Autodesk Inventor part; units mm, degrees
ref_plane "YZ Plane" through (0, 0, 0) normal (1, 0, 0) x (0, 1, 0)
ref_plane "XY Plane" through (0, 0, 0) normal (0, 0, 1) x (1, 0, 0)
sketch "Sketch1" plane through (0, 0, 0) normal (0, 1, 0) x (-1, 0, 0)
  line L0 (25.9, 0) -> (-25.9, 0)
  line L1 (0, -25.9) -> (0, 25.9)
  circle A0 centre (0, 0) radius 18.5 construction
  circle A1 centre (0, 0) radius 13 construction
  dimension "d0" = 37
  dimension "d1" = 26
sketch "Sketch2" plane through (0, 0, 0) normal (0, 1, 0) x (-1, 0, 0)
  line L0 (29.4, 0) -> (-29.4, 0)
  line L1 (0, -36.8) -> (0, 73.8)
  line L2 (-21, 58) -> (-21, -21)
  line L3 (-21, -21) -> (21, -21)
  line L4 (21, -21) -> (21, 58)
  line L5 (-21, 58) -> (21, 58)
  point P0 (0, 0)
  dimension "d3" = 42
  dimension "d29" = 21
  dimension "d30" = 58
extrude "Extrusion1" add sketch "Sketch2" along normal blind 7
sketch "Sketch6" plane through (0, 0, 0) normal (0, 1, 0) x (-1, 0, 0)
  line L0 (21, -21) -> (-21, -21)
  line L1 (21, 58) -> (21, -21)
  line L2 (-21, -21) -> (21, -21)
  line L3 (21, -21) -> (21, 58)
  line L4 (-21, 58) -> (-21, -21)
  line L5 (29.4, 0) -> (-29.4, 0)
  line L6 (0, -36.3) -> (0, 70.8)
  arc A0 (-16, 0) -> (16, 0) centre (0, 0) ccw
  line L7 (16, 0) -> (16, 58)
  line L8 (21, 58) -> (-21, 58)
  line L9 (16, 58) -> (21, 58)
  line L10 (-16, 0) -> (-16, 58)
  line L11 (-16, 58) -> (-21, 58)
  point P0 (-17.3617, -21)
  dimension "d18" = 32
extrude "Extrusion5" add sketch "Sketch6" against normal blind 5.5 contours L0 L6 A0 L5 L1 | L0 L4 L5 A0 L6 | L5 L7 L8 L1 | L4 L8 L10 L5
sketch "Sketch4" plane through (0, 0, 0) normal (0, 0, 1) x (1, 0, 0)
  line L0 (-18.5, 0) -> (18.5, 0)
  line L1 (18.5, 0) -> (18.5, -2.5)
  line L2 (18.5, -2.5) -> (-18.5, -2.5)
  line L3 (-18.5, -2.5) -> (-18.5, 0)
  line L4 (-25.9, 0) -> (25.9, 0)
  line L5 (0, -3) -> (0, 0.5)
  point P0 (0, 0)
  dimension "d10" = 37
  dimension "d11" = 2.5
extrude "Extrusion6" cut sketch "Sketch4" against normal blind 21
sketch "Sketch5" plane through (0, 0, 0) normal (0, 1, 0) x (-1, 0, 0)
  circle A0 centre (0, 0) radius 18.5 construction
  circle A1 centre (0, 0) radius 18.5 construction
  line L0 (25.9, 0) -> (-25.9, 0)
  line L1 (0, -28.9) -> (0, 26.4)
  line L2 (-18.5, -21) -> (18.5, -21)
  line L3 (18.5, -21) -> (18.5, -18.5)
  line L4 (18.5, -18.5) -> (-18.5, -18.5)
  line L5 (-18.5, -18.5) -> (-18.5, -21)
  dimension "d25" = 37
  dimension "d26" = 21
extrude "Extrusion7" add sketch "Sketch5" against normal blind 2.5
sketch "Sketch7" plane through (0, 0, 0) normal (0, 0, 1) x (1, 0, 0)
  line L0 (-18.5, 0) -> (18.5, 0)
  line L1 (18.5, 0) -> (18.5, -2.5)
  line L2 (18.5, -2.5) -> (-18.5, -2.5)
  line L3 (-18.5, -2.5) -> (-18.5, 0)
  line L4 (16, 0) -> (-16, 0)
  line L5 (-25.9, 0) -> (25.9, 0)
  line L6 (0, -3) -> (0, 0.5)
  dimension "d53" = 2.5
  dimension "d54" = 18.5
extrude "Extrusion8" cut sketch "Sketch7" along normal blind 58
sketch "Sketch8" plane through (0, 0, 0) normal (0, 1, 0) x (-1, 0, 0)
  circle A0 centre (0, 0) radius 13
  dimension "d34" = 26
extrude "Extrusion9" cut sketch "Sketch8" along normal through all
pattern_linear "Rectangular Pattern1" count 2 spacing 37 along (0, 0, 1) of "Extrusion9"
sketch "Sketch9" plane through (0, 7, 0) normal (0, 1, 0) x (1, 0, 0)
  circle A0 centre (0, 0) radius 13
  circle A1 centre (0, 0) radius 15
  dimension "d40" = 26
  dimension "d41" = 30
extrude "Extrusion10" [suppressed]
sketch "Sketch10" plane through (0, 5, 0) normal (0, 1, 0) x (1, 0, 0)
  arc A0 (16, 0) -> (-16, 0) centre (0, 0) ccw
  line L0 (1.5, -18) -> (-1.5, -18)
  line L1 (-29.4, 0) -> (29.4, 0)
  line L2 (0, 36.3) -> (0, -70.8)
  line L3 (1.5, -12) -> (-1.5, -12)
  line L4 (1.5, -12) -> (1.5, -18)
  line L5 (-1.5, -18) -> (-1.5, -12)
  dimension "d48" = 3
  dimension "d49" = 12
  dimension "d50" = 6
extrude "Extrusion11" [suppressed]
ref_plane "Work Plane1" through (0, 5, 0) normal (0, 1, 0) x (-1, 0, 0)
sketch "Sketch12" plane through (0, 5, 0) normal (0, 1, 0) x (-1, 0, 0)
  line L0 (21, 58) -> (21, -21)
  line L1 (21, -21) -> (-21, -21)
  line L2 (-21, -21) -> (-21, -51)
  line L3 (-21, -51) -> (21, -51)
  line L4 (21, -51) -> (21, -21)
  point P0 (0, 0)
  dimension "d61" = 42
  dimension "d62" = 30
extrude "Extrusion12" add sketch "Sketch12" against normal blind 34.5
sketch "Sketch13" plane through (0, 0, 0) normal (1, 0, 0) x (0, 1, 0)
  line L0 (-31.4, 0) -> (13.4, 0)
  line L1 (0, -62.5) -> (0, 32)
  line L2 (7, -19) -> (7, -49)
  line L3 (7, -49) -> (-25, -43.3575)
  line L4 (-25, -43.3575) -> (-25, -30.647)
  line L5 (7, -19) -> (-25, -30.647)
  point P0 (0, 0)
  dimension "d85" = 25
  dimension "d86" = 7
  dimension "d87" = 49
  dimension "d88" = 30
  dimension "d89" = 100
  dimension "d90" = 110
extrude "Extrusion14" cut sketch "Sketch13" along normal mid plane 38
sketch "Sketch14" plane through (0, 5, 0) normal (0, 1, 0) x (-1, 0, 0)
  line L0 (0, -72.3) -> (0, 76.8)
  line L1 (19, 56) -> (-19, 56)
  line L2 (-19, 56) -> (-19, -49)
  line L3 (-19, -49) -> (19, -49)
  line L4 (19, -49) -> (19, 56)
  line L5 (21, 58) -> (-21, 58)
  line L6 (-21, 58) -> (-21, -51)
  line L7 (-21, -51) -> (21, -51)
  line L8 (21, -51) -> (21, 58)
  line L9 (29.4, 0) -> (-29.4, 0)
  dimension "d91" = 51
  dimension "d92" = 58
  dimension "d93" = 42
  dimension "d94" = 38
  dimension "d95" = 56
  dimension "d96" = 49
extrude "Extrusion15" add sketch "Sketch14" along normal blind 8 contours L7 L6 L9 L2 L3 L0 | L0 L3 L4 L9 L8 L7 | L6 L5 L0 L1 L2 L9 | L9 L4 L1 L0 L5 L8
fillet "Fillet3" radius 2 2 edges at (21, 3.75, 58) (-21, 3.75, 58)
fillet "Fillet4" radius 2 2 edges at (16, -4, 58) (-16, -4, 58)
fillet "Fillet5" radius 2 2 edges at (21, -17.5, -21) (-21, -17.5, -21)
fillet "Fillet6" radius 2 2 edges at (0, 7, 56) (0, 7, -19)
fillet "Fillet7" radius 4 2 edges at (0, -25, -30.647) (0, -25, -43.3575)
properties part number "NespressoSpeedfiller"
Build history of the part. All positions in model axes, mm. A direction names the side the tool comes from. Round coordinates to 2 decimals unless told otherwise and drop trailing zeros. Write each loop counter-clockwise with the first axis right and the second up, starting at its lowest first coordinate (ties: lowest second). Pieces come first, ordered by that corner, then holes.
1) Band-saw the part on D-D, the plane y = 8. List the corners of the cut face in (x, z).
2) 3-axis set-ups, long thin cutter, end or side, ignore diameter. For faces 5 (the cylindrical face through (0.3, 6.6, -18.8)), 6 (the cylindrical face through (0, -4, -16)), 7 (the cylindrical face through (-20.4, -17.67, -21.57)): which of +Z, -Z, +X, -X, +Y, -Y reach the whole face in a straight line?
3) Mould opens along X. For faces 1 (the flat face through (0, 8, 58)), 2 (the flat face through (-21, 1, -10)), 3 (the cylindrical face through (20.4, 3.88, 57.43)), 4 (the flat face through (-16, -4, 28)) say: +X half, -X half, draft (parallel to the pull), parting line (faces both ways), or undercut.
4) Band-saw the part on B-B, the plane x = 0. Give the number of separate pieces and of enclosed holes in the cut face, and give its area (3 significant figures).
5) Band-saw the part on A-A, the plane z = 37. List the corners of the cut face in (x, y), and give its area (4 significant figures).
6) Drill centre lines: probe 1 along X at (y, z) = (-11, -42.5); probe 2 along X at (y, z) = (4.75, 37); probe 3 along Y at (x, z) = (-17.5, 21). Where is each one in solid material? Low to high.
7) Band-saw the part on C-C, the plane z = 22. List the corners of the cut face in (x, y).
8) Pin check, flat tips, straight feed: pin 1 (11 mm diameter, centred on x = 5.5, z = 23, fed in from +Y); pin 2 (7 mm diameter, centred on x = -0.5, z = -36, fed in from +Y); pin 3 (5 mm diameter, centred on x = 13, y = -25, fed in from +Z). Stop position of each tip, or through.
Ans:
1. outline: (-21, -51) - (21, -51) - (21, 56) arc R2 ccw to (19, 58) - (-19, 58) arc R2 ccw to (-21, 56) - close; hole (-19, -49) - (19, -49) - (19, 55.73) - (-19, 55.73) - close
2. face 5: +Y
2. face 6: +Z, -Y
2. face 7: +Z, -X, -Y
3. face 1: draft
3. face 2: -X half
3. face 3: +X half
3. face 4: undercut
4. separate pieces: 3
4. enclosed holes: 0
4. area: 650 mm2
5. outline: (-21, -5.5) - (-16, -5.5) - (-16, -2.5) - (-18.5, -2.5) - (-18.5, 0) - (-13, 0) - (-13, 7) - (-19, 7) - (-19, 13) - (-21, 13) - close; (13, 0) - (18.5, 0) - (18.5, -2.5) - (16, -2.5) - (16, -5.5) - (21, -5.5) - (21, 13) - (19, 13) - (19, 7) - (13, 7) - close
5. area: 178.5 mm2
6. probe 1: x = -21 to -19, 19 to 21
6. probe 2: x = -21 to -13, 13 to 21
6. probe 3: y = -5.5 to -2.5, 0 to 7
7. outline: (-21, -5.5) - (-16, -5.5) - (-16, -2.5) - (-18.5, -2.5) - (-18.5, 0) - (18.5, 0) - (18.5, -2.5) - (16, -2.5) - (16, -5.5) - (21, -5.5) - (21, 13) - (19, 13) - (19, 7) - (-19, 7) - (-19, 13) - (-21, 13) - close
8. pin 1: stops at y = 7
8. pin 2: stops at y = -24.89
8. pin 3: stops at z = -21
